Read the model definition and answer for the solid it produces. Units are mm, in the model's axes. A direction names the side the tool comes from. Round coordinates to 2 decimals unless told otherwise and drop trailing zeros. Loops run counter-clockwise (first coordinate to the right, second up) from the corner with the lowest first, then second, coordinate; pieces in that order, holes last. Notation, with made-up numbers: M 69,73 L 124,73 A21 cw 124,83 Z; hole C -1.75,27.5 d1. An arc over 180 degrees is marked long. Write each question's results on one line, items separated by ' | '.
from build123d import *

# Parameters (mm, degrees)
SKETCH1_W           = 28
SKETCH1_H           = 28
BOSS_EXTRUDE1_DEPTH = 3.25
SKETCH2_R           = 5
BOSS_EXTRUDE2_DEPTH = 16
SKETCH3_R           = 1.6
CUT_EXTRUDE1_DEPTH  = 45.029109689
FILLET1_R           = 0.5
SKETCH4_W           = 13
SKETCH4_H           = 2.5
SKETCH4_W_2         = 2.5
SKETCH4_H_2         = 13
BOSS_EXTRUDE3_DEPTH = 0.5


with BuildPart() as part:
    # Sketch1 → Boss-Extrude1 (new body)
    with BuildSketch(Plane.XY):
        with Locations((14, 14)):
            Rectangle(SKETCH1_W, SKETCH1_H)
    extrude(amount=BOSS_EXTRUDE1_DEPTH)

    # Sketch2 → Boss-Extrude2 (add)
    with BuildSketch(Plane.XY.offset(3.25)):
        with Locations((14, 14)):
            Circle(SKETCH2_R)
    extrude(amount=BOSS_EXTRUDE2_DEPTH)

    # Sketch3 → Cut-Extrude1 (cut, through all)
    with BuildSketch(Plane(origin=(0, 0, 0), x_dir=(-1, 0, 0), z_dir=(0, 0, -1))):
        with Locations((-24, 24)):
            Circle(SKETCH3_R)
        with Locations((-4, 24)):
            Circle(SKETCH3_R)
        with Locations((-4, 4)):
            Circle(SKETCH3_R)
        with Locations((-24, 4)):
            Circle(SKETCH3_R)
    extrude(amount=-CUT_EXTRUDE1_DEPTH, mode=Mode.SUBTRACT)

    # Fillet1
    fillet1_edges = [part.edges().sort_by_distance(p)[0] for p in [
        (9, 14, 19.25),
    ]]
    fillet(fillet1_edges, radius=FILLET1_R)

    # Sketch4 → Boss-Extrude3 (add)
    with BuildSketch(Plane(origin=(0, 0, 0), x_dir=(-1, 0, 0), z_dir=(0, 0, -1))):
        with Locations((-14, 24.25)):
            Rectangle(SKETCH4_W, SKETCH4_H)
        with Locations((-3.75, 14)):
            Rectangle(SKETCH4_W_2, SKETCH4_H_2)
        with Locations((-14, 3.75)):
            Rectangle(SKETCH4_W, SKETCH4_H)
        with Locations((-24.25, 14)):
            Rectangle(SKETCH4_W_2, SKETCH4_H_2)
    extrude(amount=BOSS_EXTRUDE3_DEPTH)


solid = part.part
Item 1: Straight lines are drawn through the part: line 1 (Y direction, x = 24, z = 1.9); line 2 (Z direction, x = 9.25, y = 6.5); line 3 (Z direction, x = 13.25, y = 11.5). For each, find the intervals that lie inside material, in ascending order.
Outcome:
line 1: y = 0 to 2.4, 5.6 to 22.4, 25.6 to 28 | line 2: z = 0 to 3.25 | line 3: z = 0 to 19.25
Item 2: The part is cut by section B-B (x = 14). Determine the outline of the cut face in (y, z).
Outcome:
outline: M 0,0 L 2.5,0 L 2.5,-0.5 L 5,-0.5 L 5,0 L 23,0 L 23,-0.5 L 25.5,-0.5 L 25.5,0 L 28,0 L 28,3.25 L 19,3.25 L 19,18.75 A0.5 ccw 18.5,19.25 L 9.5,19.25 A0.5 ccw 9,18.75 L 9,3.25 L 0,3.25 Z
Item 3: The part is cut by section A-A (x = 24). Determine the outline of the cut face in (y, z).
Outcome:
outline: M 0,0 L 2.4,0 L 2.4,3.25 L 0,3.25 Z; M 5.6,0 L 7.5,0 L 7.5,-0.5 L 20.5,-0.5 L 20.5,0 L 22.4,0 L 22.4,3.25 L 5.6,3.25 Z; M 25.6,0 L 28,0 L 28,3.25 L 25.6,3.25 Z
Item 4: For faces 5 (the face through (28, 14, 2)), 6 (the face through (8, 14, 3.25)), determine the directions among +Z, -Z, +X, -X, +Y, -Y from which every point of the face is accessible in a straight line to the end or side of a thin tool.
Outcome:
face 5: +Z, -Z, +X, +Y, -Y | face 6: +Z
Item 5: The part is cut by section C-C (z = 6). Determine the outline of the cut face in (x, y), plus the area to 3 significant figures.
Outcome:
outline: C 14,14 d10 | area: 78.5 mm2
Item 6: Flat-ended cylindrical pins translate along their axes: pin 1 (5 mm diameter, centred on y = 17, z = 12, fed in from +X); pin 2 (0.6 mm diameter, centred on y = 24, z = -0.5, fed in from -X); pin 3 (5 mm diameter, centred on x = 4, y = 24, fed in from +Z). Find the tip coordinate at first contact, or state that the pin passes through.
Outcome:
pin 1: stops at x = 18.97 | pin 2: stops at x = 7.5 | pin 3: stops at z = 3.25
Item 7: The mould has two halves that part along X. Classify faces 1 (the face through (24, 14, -0.5)), 2 (the face through (0, 14, 2)), 3 (the face through (24.208, 25.586, 1.602)), 4 (the face through (5.27, 3.03, 1.6)): pulls with the +X half, pulls with the -X half, needs draft (parallel to the pull), parting line crosses it, or undercut.
Outcome:
face 1: needs draft | face 2: pulls with the -X half | face 3: undercut | face 4: undercut
